Autodesk Inventor part; units mm, degrees
ref_plane "YZ Plane" through (0, 0, 0) normal (1, 0, 0) x (0, 1, 0)
ref_plane "XZ Plane" through (0, 0, 0) normal (0, 1, 0) x (-1, 0, 0)
ref_plane "XY Plane" through (0, 0, 0) normal (0, 0, 1) x (1, 0, 0)
sketch "Sketch1" plane through (0, 0, 0) normal (0, 0, 1) x (1, 0, 0)
  arc A0 (12.7, 228.2469) -> (-12.7, 228.2469) centre (0, 0) ccw
  line L0 (-25.4, 188.7991) -> (-12.7, 228.2469)
  line L1 (12.7, 228.2469) -> (25.4, 188.7991)
  arc A1 (-58.4538, 221.0003) -> (-82.6106, 213.1512) centre (0, 0) ccw
  line L2 (-82.499, 171.7096) -> (-82.6106, 213.1512)
  line L3 (-58.4538, 221.0003) -> (-34.1853, 187.4076)
  arc A2 (-123.8857, 192.1205) -> (-144.4347, 177.1908) centre (0, 0) ccw
  line L4 (-131.5223, 137.8119) -> (-144.4347, 177.1908)
  line L5 (-123.8857, 192.1205) -> (-90.4243, 167.6714)
  arc A3 (-177.1908, 144.4347) -> (-192.1205, 123.8857) centre (0, 0) ccw
  line L6 (-167.6714, 90.4243) -> (-192.1205, 123.8857)
  line L7 (-177.1908, 144.4347) -> (-137.8119, 131.5223)
  arc A4 (-213.1512, 82.6106) -> (-221.0003, 58.4538) centre (0, 0) ccw
  line L8 (-187.4076, 34.1853) -> (-221.0003, 58.4538)
  line L9 (-213.1512, 82.6106) -> (-171.7096, 82.499)
  arc A5 (-228.2469, 12.7) -> (-228.2469, -12.7) centre (0, 0) ccw
  line L10 (-188.7991, -25.4) -> (-228.2469, -12.7)
  line L11 (-228.2469, 12.7) -> (-188.7991, 25.4)
  arc A6 (-221.0003, -58.4538) -> (-213.1512, -82.6106) centre (0, 0) ccw
  line L12 (-171.7096, -82.499) -> (-213.1512, -82.6106)
  line L13 (-221.0003, -58.4538) -> (-187.4076, -34.1853)
  arc A7 (-192.1205, -123.8857) -> (-177.1908, -144.4347) centre (0, 0) ccw
  line L14 (-137.8119, -131.5223) -> (-177.1908, -144.4347)
  line L15 (-192.1205, -123.8857) -> (-167.6714, -90.4243)
  arc A8 (-144.4347, -177.1908) -> (-123.8857, -192.1205) centre (0, 0) ccw
  line L16 (-90.4243, -167.6714) -> (-123.8857, -192.1205)
  line L17 (-144.4347, -177.1908) -> (-131.5223, -137.8119)
  arc A9 (-82.6106, -213.1512) -> (-58.4538, -221.0003) centre (0, 0) ccw
  line L18 (-34.1853, -187.4076) -> (-58.4538, -221.0003)
  line L19 (-82.6106, -213.1512) -> (-82.499, -171.7096)
  arc A10 (-12.7, -228.2469) -> (12.7, -228.2469) centre (0, 0) ccw
  line L20 (25.4, -188.7991) -> (12.7, -228.2469)
  line L21 (-12.7, -228.2469) -> (-25.4, -188.7991)
  arc A11 (58.4538, -221.0003) -> (82.6106, -213.1512) centre (0, 0) ccw
  line L22 (82.499, -171.7096) -> (82.6106, -213.1512)
  line L23 (58.4538, -221.0003) -> (34.1853, -187.4076)
  arc A12 (123.8857, -192.1205) -> (144.4347, -177.1908) centre (0, 0) ccw
  line L24 (131.5223, -137.8119) -> (144.4347, -177.1908)
  line L25 (123.8857, -192.1205) -> (90.4243, -167.6714)
  arc A13 (177.1908, -144.4347) -> (192.1205, -123.8857) centre (0, 0) ccw
  line L26 (167.6714, -90.4243) -> (192.1205, -123.8857)
  line L27 (177.1908, -144.4347) -> (137.8119, -131.5223)
  arc A14 (213.1512, -82.6106) -> (221.0003, -58.4538) centre (0, 0) ccw
  line L28 (187.4076, -34.1853) -> (221.0003, -58.4538)
  line L29 (213.1512, -82.6106) -> (171.7096, -82.499)
  arc A15 (228.2469, -12.7) -> (228.2469, 12.7) centre (0, 0) ccw
  line L30 (188.7991, 25.4) -> (228.2469, 12.7)
  line L31 (228.2469, -12.7) -> (188.7991, -25.4)
  arc A16 (221.0003, 58.4538) -> (213.1512, 82.6106) centre (0, 0) ccw
  line L32 (171.7096, 82.499) -> (213.1512, 82.6106)
  line L33 (221.0003, 58.4538) -> (187.4076, 34.1853)
  arc A17 (192.1205, 123.8857) -> (177.1908, 144.4347) centre (0, 0) ccw
  line L34 (137.8119, 131.5223) -> (177.1908, 144.4347)
  line L35 (192.1205, 123.8857) -> (167.6714, 90.4243)
  arc A18 (144.4347, 177.1908) -> (123.8857, 192.1205) centre (0, 0) ccw
  line L36 (90.4243, 167.6714) -> (123.8857, 192.1205)
  line L37 (144.4347, 177.1908) -> (131.5223, 137.8119)
  arc A19 (82.6106, 213.1512) -> (58.4538, 221.0003) centre (0, 0) ccw
  line L38 (34.1853, 187.4076) -> (58.4538, 221.0003)
  line L39 (82.6106, 213.1512) -> (82.499, 171.7096)
  arc A20 (-131.5223, 137.8119) -> (-137.8119, 131.5223) centre (0, 0) ccw
  arc A21 (-167.6714, 90.4243) -> (-171.7096, 82.499) centre (0, 0) ccw
  arc A22 (-187.4076, 34.1853) -> (-188.7991, 25.4) centre (0, 0) ccw
  arc A23 (-188.7991, -25.4) -> (-187.4076, -34.1853) centre (0, 0) ccw
  arc A24 (-171.7096, -82.499) -> (-167.6714, -90.4243) centre (0, 0) ccw
  arc A25 (-82.499, 171.7096) -> (-90.4243, 167.6714) centre (0, 0) ccw
  arc A26 (-25.4, 188.7991) -> (-34.1853, 187.4076) centre (0, 0) ccw
  arc A27 (34.1853, 187.4076) -> (25.4, 188.7991) centre (0, 0) ccw
  arc A28 (90.4243, 167.6714) -> (82.499, 171.7096) centre (0, 0) ccw
  arc A29 (137.8119, 131.5223) -> (131.5223, 137.8119) centre (0, 0) ccw
  arc A30 (171.7096, 82.499) -> (167.6714, 90.4243) centre (0, 0) ccw
  arc A31 (188.7991, 25.4) -> (187.4076, 34.1853) centre (0, 0) ccw
  arc A32 (187.4076, -34.1853) -> (188.7991, -25.4) centre (0, 0) ccw
  arc A33 (167.6714, -90.4243) -> (171.7096, -82.499) centre (0, 0) ccw
  arc A34 (131.5223, -137.8119) -> (137.8119, -131.5223) centre (0, 0) ccw
  arc A35 (82.499, -171.7096) -> (90.4243, -167.6714) centre (0, 0) ccw
  arc A36 (-137.8119, -131.5223) -> (-131.5223, -137.8119) centre (0, 0) ccw
  arc A37 (-90.4243, -167.6714) -> (-82.499, -171.7096) centre (0, 0) ccw
  arc A38 (-34.1853, -187.4076) -> (-25.4, -188.7991) centre (0, 0) ccw
  arc A39 (25.4, -188.7991) -> (34.1853, -187.4076) centre (0, 0) ccw
  circle A40 centre (0, 0) radius 75
  dimension "d10" = 457.2
  dimension "d18" = 360
  dimension "d20" = 150
extrude "Extrusion1" add sketch "Sketch1" along normal blind 50.8
properties part number "Engrenagem"
CAD build for the part. Positions are in the model's coordinates, mm. A direction names the side the tool comes from. Round coordinates to 2 decimals unless told otherwise and drop trailing zeros. Order: outer loops, then holes, each group sorted by start corner. A loop starts at its lowest first (then second) coordinate and runs counter-clockwise, first axis right, second up. Notation, with made-up numbers: (-36.75, 52.5) - (-2.75, 52.5) arc R12 ccw to (-2.75, 71.5) - close; hole circle Ø10 at (67, 82). An arc over 180 degrees is marked (long way). Return JSON: item names as keys, results as strings.
(1) Cut at D-D (y = -154). Give the cut face in (x, z), then the cut area to 3 significant figures.
Answer key:
{"outline": "(-136.83, 0) - (136.83, 0) - (136.83, 50.8) - (-136.83, 50.8) - close", "area": "13,900 mm^2"}
(2) Pin check, flat tips, straight feed: pin 1 Ø8 at (x, z) = (-126.5, 6) entering from +Y; pin 2 Ø1.5 at (x, z) = (141.5, 20.5) entering from -Y; pin 3 Ø2 at (x, y) = (-55.5, -81.5) entering from -Z; pin 4 Ø12 at (y, z) = (-105, 13.5) entering from +X. Stop position of each tip, or through.
Answer key:
{"pin 1": "stops at y = 192.12", "pin 2": "stops at y = -180.13", "pin 3": "stops at z = 0", "pin 4": "stops at x = 182.71"}
(3) Tool access for faces 1 (the face through (-203.97, 46.15, 25.04)), 2 (the face through (46.15, 203.97, 25.04)), 3 (the face through (134.22, 185.05, 25.04)), 4 (the face through (-157.23, -137.89, 25.04)): list every direction of +Z, -Z, +X, -X, +Y, -Y with a clear straight run to the whole face (end or side of a thin tool).
Answer key:
{"face 1": "+Z, -Z, -X", "face 2": "+Z, -Z, +Y", "face 3": "+Z, -Z, +X, +Y", "face 4": "+Z, -Z"}
(4) Pull direction X, two halves, no side cores. Call faces 5 (the face through (217.466, -70.472, 25.044)), 6 (the face through (-180.07, -107.39, 25.04)), 7 (the face through (-106.921, -179.725, 25.044)), 8 (the face through (106.921, 179.725, 25.044)): +X half, -X half, draft (parallel to the pull), parting line (faces both ways), or undercut.
Answer key:
{"face 5": "+X half", "face 6": "-X half", "face 7": "undercut", "face 8": "undercut"}
(5) Wall check: probe 1 along X at (y, z) = (-206.5, 6); probe 2 along Y at (x, z) = (-169.5, 25); probe 3 along X at (y, z) = (69, 8). Give the ranges that are in metal, low to high. Write a range as from..to.
Answer key:
{"probe 1": "x = -82.59..-47.98, -19.7..19.7, 47.98..82.59", "probe 2": "y = -141.91..-92.93, -86.95..86.95, 92.93..141.91", "probe 3": "x = -217.94..-29.39, 29.39..217.94"}
(6) Cut at C-C (y = 199). Give the cut face in (x, z).
Answer key:
{"outline": "(-82.57, 0) - (-42.56, 0) - (-42.56, 50.8) - (-82.57, 50.8) - close; (-22.12, 0) - (22.12, 0) - (22.12, 50.8) - (-22.12, 50.8) - close; (42.56, 0) - (82.57, 0) - (82.57, 50.8) - (42.56, 50.8) - close"}
(7) Cut at A-A (x = 0). Give the cut face in (y, z), then the cut area to 3 significant figures.
Answer key:
{"outline": "(-228.6, 0) - (-75, 0) - (-75, 50.8) - (-228.6, 50.8) - close; (75, 0) - (228.6, 0) - (228.6, 50.8) - (75, 50.8) - close", "area": "15,600 mm^2"}
